Design review of the part built by this model. Coordinates are the model's own, in mm. Coordinates: 2 decimals unless noted, no trailing zeros. Write each loop counter-clockwise with the first axis right and the second up, starting at its lowest first coordinate (ties: lowest second). Pieces come first, ordered by that corner, then holes.
Q1. Clearance check with a flat-ended pin moving along its axis: pin 1 Ø4 at (x, z) = (-44.135, 89) entering from -Y. State where the tip first meets the part, or that it passes through.
Q2. To check wall thickness, follow probe 1 along X at (y, z) = (1.85, 89) (3 decimals); probe 2 along X at (y, z) = (2.5, -4.5); probe 3 along X at (y, z) = (2.4, -82.5). State the ranges of each line that lie inside material, in increasing order.
Q3. Add section D-D, the plane x = -80. Give the boundary of the cut face in (y, z), plus the area to 3 significant figures.
Q4. Add section C-C, the plane y = 1.5. Give the number of separate pieces and of enclosed holes in the cut face, plus the area to 3 significant figures.
Q5. Add section B-B, the plane x = 0. Give the boundary of the cut face in (y, z), plus the area to 3 significant figures.
Q6. Add section A-A, the plane z = 0. Give the boundary of the cut face in (x, y).
from build123d import *

# Parameters (mm, degrees)
SKETCH_1_R                   = 145
EXTRUDE_1_DEPTH              = 3
SKETCH_2_R                   = 2.5
CUT_EXTRUDE_1_DEPTH          = 10
PATTERN_CIRCULAR_1_OUTLINE_R = 2.5
PATTERN_CIRCULAR_1_DEPTH     = 3
SKETCH_5_W                   = 50
SKETCH_5_H                   = 30
CUT_EXTRUDE_2_DEPTH          = 10
FILLET_1_R                   = 5


# Read off the part's stored shape, not the designer's step: 阵列(圆周)1
with BuildPart() as part:
    # 草图1 → 凸台-拉伸1 (new body)
    with BuildSketch(Plane(origin=(0, 0, 0), x_dir=(1, 0, 0), z_dir=(0, 1, 0))):
        with Locations(Location((0, 0, 0), (0, 0, 270))):
            Circle(SKETCH_1_R)
    extrude(amount=EXTRUDE_1_DEPTH)

    # 草图2 → 切除-拉伸1 (cut)
    with BuildSketch(Plane(origin=(0, 3, 0), x_dir=(1, 0, 0), z_dir=(0, 1, 0))):
        with Locations(Location((-44.135, -89, 0), (0, 0, 270))):
            Circle(SKETCH_2_R)
        with Locations(Location((-44.135, -130, 0), (0, 0, 270))):
            Circle(SKETCH_2_R)
    cut_extrude_1 = extrude(amount=-CUT_EXTRUDE_1_DEPTH, mode=Mode.SUBTRACT)

    # 镜向1: 切除-拉伸1 across plane
    add(cut_extrude_1.mirror(Plane(origin=(0, 0, 0), x_dir=(0, 0, 1), z_dir=(1, 0, 0))), mode=Mode.SUBTRACT)

    # 阵列(圆周)1 outline → 阵列(圆周)1 (cut)
    with BuildSketch(Plane(origin=(0, 0, 0), x_dir=(1, 0, 0), z_dir=(0, 1, 0))):
        with Locations((55.121653534, 82.91756691)):
            Circle(PATTERN_CIRCULAR_1_OUTLINE_R)
        with Locations((90.628695089, 103.41756691)):
            Circle(PATTERN_CIRCULAR_1_OUTLINE_R)
        with Locations((-99.256653534, 6.473504518)):
            Circle(PATTERN_CIRCULAR_1_OUTLINE_R)
        with Locations((-134.763695089, 26.973504518)):
            Circle(PATTERN_CIRCULAR_1_OUTLINE_R)
        with Locations((99.239525897, 6.352725277)):
            Circle(PATTERN_CIRCULAR_1_OUTLINE_R)
        with Locations((-90.532661016, 103.342344321)):
            Circle(PATTERN_CIRCULAR_1_OUTLINE_R)
        with Locations((-55.025619461, 82.842344321)):
            Circle(PATTERN_CIRCULAR_1_OUTLINE_R)
        with Locations((134.746567453, 26.852725277)):
            Circle(PATTERN_CIRCULAR_1_OUTLINE_R)
    extrude(amount=PATTERN_CIRCULAR_1_DEPTH, mode=Mode.SUBTRACT)

    # 草图5 → 切除-拉伸2 (cut)
    with BuildSketch(Plane(origin=(0, 3, 0), x_dir=(1, 0, 0), z_dir=(0, 1, 0))):
        Rectangle(SKETCH_5_W, SKETCH_5_H)
    extrude(amount=-CUT_EXTRUDE_2_DEPTH, mode=Mode.SUBTRACT)

    # 圆角1
    fillet_1_edges = [part.edges().sort_by_distance(p)[0] for p in [
        (25, 1.5, -15),
        (25, 1.5, 15),
        (-25, 1.5, 15),
        (-25, 1.5, -15),
    ]]
    fillet(fillet_1_edges, radius=FILLET_1_R)


solid = part.part
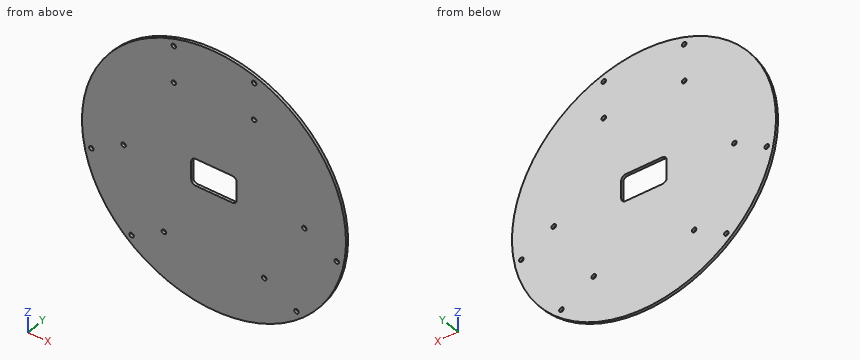
Here are the results:
1. pin 1: passes through
2. probe 1: x = -114.473 to -46.635, -41.635 to 41.635, 46.635 to 114.473
2. probe 2: x = -144.93 to -100.79, -97.72 to -25, 25 to 97.56, 100.92 to 144.93
2. probe 3: x = -119.24 to -57.5, -52.55 to 52.66, 57.59 to 119.24
3. outline: (0, -120.93) - (3, -120.93) - (3, 120.93) - (0, 120.93) - close
3. area: 726 mm2
4. separate pieces: 1
4. enclosed holes: 13
4. area: 64,300 mm2
5. outline: (0, -145) - (3, -145) - (3, -15) - (0, -15) - close; (0, 15) - (3, 15) - (3, 145) - (0, 145) - close
5. area: 780 mm2
6. outline: (-145, 0) - (-25, 0) - (-25, 3) - (-145, 3) - close; (25, 0) - (145, 0) - (145, 3) - (25, 3) - close
